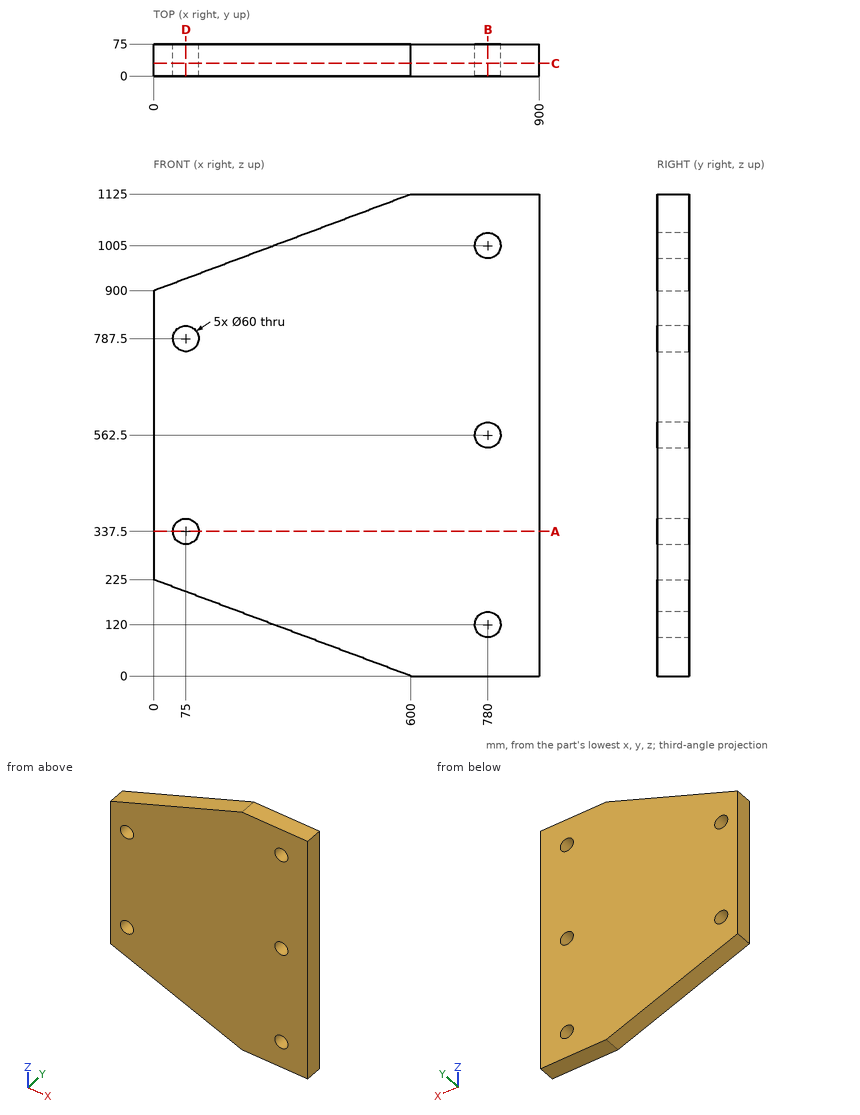
Answer from the drawing. Dimensions are ordinates in mm from the lowest x, y and z of the part. Give positions to 0.01 mm unless a question says otherwise; leave off trailing zeros. Order: outer loops, then holes, each group sorted by start corner. A loop starts at its lowest first (then second) coordinate and runs counter-clockwise, first axis right, second up.
Item 1: The part is cut by section A-A, the plane z = 337.5. Give the vertices of the cut face in (x, y).
From the geometry:
outline: (0, 0) - (45, 0) - (45, 75) - (0, 75) - close; (105, 0) - (900, 0) - (900, 75) - (105, 75) - close
Item 2: The part is cut by section D-D, the plane x = 75. Give the vertices of the cut face in (y, z) (3 decimals).
From the geometry:
outline: (0, 196.875) - (75, 196.875) - (75, 307.5) - (0, 307.5) - close; (0, 367.5) - (75, 367.5) - (75, 757.5) - (0, 757.5) - close; (0, 817.5) - (75, 817.5) - (75, 928.125) - (0, 928.125) - close
Item 3: The part is cut by section C-C, the plane y = 30. Give the vertices of the cut face in (x, z), and give its area (3 significant figures).
From the geometry:
outline: (0, 225) - (600, 0) - (900, 0) - (900, 1125) - (600, 1125) - (0, 900) - close; hole circle Ø60 at (75, 337.5); hole circle Ø60 at (75, 787.5); hole circle Ø60 at (780, 120); hole circle Ø60 at (780, 562.5); hole circle Ø60 at (780, 1005)
area: 863,000 mm2
Item 4: Given pin 1 Ø12 at (x, y) = (528, 60) entering from -Z, flat-ended and moving along its own axis, determine where the tip first touches the part or whether it passes through.
From the geometry:
pin 1: stops at z = 24.75
Item 5: Find the intervals of material crossed by probe 1 along Z at (x, y) = (760, 6); probe 2 along X at (y, z) = (27, 320); probe 3 along X at (y, z) = (63, 773.5), in increasing order.
From the geometry:
probe 1: z = 0 to 97.64, 142.36 to 540.14, 584.86 to 982.64, 1027.36 to 1125
probe 2: x = 0 to 50.63, 99.37 to 900
probe 3: x = 0 to 48.47, 101.53 to 900
Item 6: The part is cut by section B-B, the plane x = 780. Give the vertices of the cut face in (y, z).
From the geometry:
outline: (0, 0) - (75, 0) - (75, 90) - (0, 90) - close; (0, 150) - (75, 150) - (75, 532.5) - (0, 532.5) - close; (0, 592.5) - (75, 592.5) - (75, 975) - (0, 975) - close; (0, 1035) - (75, 1035) - (75, 1125) - (0, 1125) - close
